from build123d import *

# Parameters (mm, degrees)
ESQUISSE1_W             = 69.3
ESQUISSE1_H             = 32.6
ESQUISSE1_W_2           = 65.3
ESQUISSE1_H_2           = 28.6
BOSS_EXTRU_1_DEPTH      = 30
ESQUISSE3_W             = 69.3
ESQUISSE3_H             = 32.6
BOSS_EXTRU_2_DEPTH      = 2
ESQUISSE4_W             = 4
ESQUISSE4_H             = 13
ENL_V_MAT_EXTRU_1_DEPTH = 18
ENL_V_MAT_EXTRU_2_DEPTH = 18


with BuildPart() as part:
    # Esquisse1 → Boss.-Extru.1 (new body)
    with BuildSketch(Plane.XY):
        with Locations((8.234452659, -4.576404494)):
            Rectangle(ESQUISSE1_W, ESQUISSE1_H)
        with Locations((8.234452659, -4.576404494)):
            Rectangle(ESQUISSE1_W_2, ESQUISSE1_H_2, mode=Mode.SUBTRACT)
    extrude(amount=BOSS_EXTRU_1_DEPTH)

    # Esquisse3 → Boss.-Extru.2 (add)
    with BuildSketch(Plane(origin=(0, 0, 0), x_dir=(-1, 0, 0), z_dir=(0, 0, -1))):
        with Locations((-8.234452659, -4.576404494)):
            Rectangle(ESQUISSE3_W, ESQUISSE3_H)
    extrude(amount=BOSS_EXTRU_2_DEPTH)

    # Esquisse4 → Enlèv. mat.-Extru.1 (cut)
    with BuildSketch(Plane(origin=(-24.415547341, 0, 0), x_dir=(0, 0, -1), z_dir=(1, 0, 0))):
        with Locations((-2, -6.776404494)):
            Rectangle(ESQUISSE4_W, ESQUISSE4_H)
    extrude(amount=-ENL_V_MAT_EXTRU_1_DEPTH, mode=Mode.SUBTRACT)

    # Esquisse5 → Enlèv. mat.-Extru.2 (cut)
    with BuildSketch(Plane.ZY.offset(-40.884452659)):
        with BuildLine():
            Line((0, 3.111294122), (0, -7.052256907))
            ThreePointArc((0, -7.052256907), (5.081775514, -1.970481392), (0, 3.111294122))
        make_face()
    extrude(amount=-ENL_V_MAT_EXTRU_2_DEPTH, mode=Mode.SUBTRACT)


solid = part.part
Part model, mm, in its own coordinate system. A direction names the side the tool comes from. Coordinates: 2 decimals unless noted, no trailing zeros. Order: outer loops, then holes, each group sorted by start corner. A loop starts at its lowest first (then second) coordinate and runs counter-clockwise, first axis right, second up.
(1) Slice it at B-B, the plane y = 2. Write the cut outline in (x, z), and give its area (3 significant figures).
Check sheet entries:
outline: (-26.42, -2) - (42.88, -2) - (42.88, 0) - (-24.42, 0) - (-24.42, 30) - (-26.42, 30) - close; (40.88, 3.17) - (42.88, 3.17) - (42.88, 30) - (40.88, 30) - close
area: 252 mm2
(2) Probe L1, parallel to X at y = 0, z = 5; L2, parallel to Y at x = -10.5, z = 13; L3, parallel to Z at x = 32.5, y = -6. List the from-to ranges inside material, lowest first.
Check sheet entries:
L1: x = -26.42 to -24.42, 40.88 to 42.88
L2: y = -20.88 to -18.88, 9.72 to 11.72
L3: z = -2 to 0
(3) Slice it at C-C, the plane x = 10. Write the cut outline in (y, z).
Check sheet entries:
outline: (-20.88, -2) - (11.72, -2) - (11.72, 30) - (9.72, 30) - (9.72, 0) - (-18.88, 0) - (-18.88, 30) - (-20.88, 30) - close
(4) Tool access for faces 5 (the face through (8, -20, 30)), 6 (the face through (8, 9.724, 15)), 7 (the face through (-25, -0.276, 2)), 8 (the face through (-25, -7, 4)): list every direction of +Z, -Z, +X, -X, +Y, -Y with a clear straight run to the whole face (end or side of a thin tool).
Check sheet entries:
face 5: +Z, +X, -X, +Y, -Y
face 6: +Z
face 7: +X, -X
face 8: -X
(5) Pin check, flat tip, straight feed: pin 1 Ø14.5 at (x, y) = (24.5, -3) entering from +Z. Stop position of the tip, or through.
Check sheet entries:
pin 1: stops at z = 0
(6) Slice it at D-D, the plane y = -2.5. Write the cut outline in (x, z).
Check sheet entries:
outline: (-26.42, -2) - (42.88, -2) - (42.88, 0) - (-26.42, 0) - close; (-26.42, 4) - (-24.42, 4) - (-24.42, 30) - (-26.42, 30) - close; (40.88, 5.05) - (42.88, 5.05) - (42.88, 30) - (40.88, 30) - close
(7) Slice it at A-A, the plane z = 2.5. Write the cut outline in (x, y), and give its area (3 significant figures).
Check sheet entries:
outline: (-26.42, -20.88) - (42.88, -20.88) - (42.88, -6.39) - (40.88, -6.39) - (40.88, -18.88) - (-24.42, -18.88) - (-24.42, -13.28) - (-26.42, -13.28) - close; (-26.42, -0.28) - (-24.42, -0.28) - (-24.42, 9.72) - (40.88, 9.72) - (40.88, 2.45) - (42.88, 2.45) - (42.88, 11.72) - (-26.42, 11.72) - close
area: 348 mm2
(8) Pull direction X, two halves, no side cores. Call faces 1 (the face through (40.884, -5, 15)), 2 (the face through (42.884, -5, 14)), 3 (the face through (-26.416, -5, 14)), 4 (the face through (41.87, -2.08, 5.08)): pulls with the +X half, pulls with the -X half, needs draft (parallel to the pull), parting line crosses it, or undercut.
Check sheet entries:
face 1: undercut
face 2: pulls with the +X half
face 3: pulls with the -X half
face 4: needs draft
